The model under review builds one solid part; all positions refer to its coordinate system, in mm. Coordinates: 2 decimals unless noted, no trailing zeros. Loops run counter-clockwise (first coordinate to the right, second up) from the corner with the lowest first, then second, coordinate; pieces in that order, holes last. Notation, with made-up numbers: (73.5, 46.5) - (93.5, 46.5) arc R18 ccw to (93.5, 61.5) - close; hole circle Ø11 at (-31.75, -31.5). An arc over 180 degrees is marked (long way). Answer in a Markdown table with one row per item. Add a question column.
(1) We need section A-A on y = 108.5. Write out the cut boundary in (x, z).
(2) For P1, Ø6, axis at x = -1, y = 113.5, coming from the +Z side; P2, Ø1.5, axis at y = 102.5, z = -5.5, coming from the +X side; P3, Ø8, axis at y = 82, z = 4.5, coming from the +X side; P4, Ø8, axis at x = 0, z = 0, coming from the -Y side, all flat-tipped, find the tip position at first contact; note any pin that passes through.
(3) We need section B-B on y = 37. Write out the cut boundary in (x, z).
(4) For line 1 along X through (y, z) = (10.5, 0); line 2 along Y through (x, z) = (-6, 2.25); line 3 along Z through (x, y) = (2.5, 11), list the stretches that pass through material, from the lowest coordinate up.
(5) Mouldability with a two-part tool opening along X and no side actions: class faces 1 (the cylindrical face through (0.59, 7.6, 4.46)), 2 (the flat face through (-3, 98.298, 3)), 3 (the cylindrical face through (-3.843, 113.951, -0.853)), 4 (the conical face through (-0.169, 17.234, -0.763)) as +X half, -X half, draft (parallel to the pull), parting line (faces both ways), or undercut.
from build123d import *

# Parameters (mm, degrees)
SKETCH1_R                  = 7.14375
BOSS_EXTRUDE1_DEPTH        = 130.048
M10X1_0_TAPPED_HOLE1_D     = 9
M10X1_0_TAPPED_HOLE1_DEPTH = 15
M10X1_0_TAPPED_HOLE1_TIP   = 2.703872786
CUT_EXTRUDE1_START         = -31.75
SKETCH4_R                  = 7.14375
SKETCH4_R_2                = 3.937
CUT_EXTRUDE1_DEPTH         = 31.75


with BuildPart() as part:
    # Sketch1 → Boss-Extrude1 (new body)
    with BuildSketch(Plane(origin=(0, 0, 0), x_dir=(1, 0, 0), z_dir=(0, 1, 0))):
        with Locations(Location((0, 0, 0), (0, 0, 270))):
            Circle(SKETCH1_R)
    extrude(amount=BOSS_EXTRUDE1_DEPTH)

    # M10x1.0 Tapped Hole1
    with Locations(Plane.XZ):
        with Locations((0, 0)):
            Hole(M10X1_0_TAPPED_HOLE1_D / 2, depth=M10X1_0_TAPPED_HOLE1_DEPTH)
            with Locations((0, 0, -(M10X1_0_TAPPED_HOLE1_DEPTH + M10X1_0_TAPPED_HOLE1_TIP / 2))):  # 118° drill point
                Cone(0, M10X1_0_TAPPED_HOLE1_D / 2, M10X1_0_TAPPED_HOLE1_TIP, mode=Mode.SUBTRACT)

    # Sketch4 → Cut-Extrude1 (cut)
    with BuildSketch(Plane(origin=(0, 130.048, 0), x_dir=(1, 0, 0), z_dir=(0, 1, 0)).offset(CUT_EXTRUDE1_START)):
        with Locations(Location((0, 0, 0), (0, 0, 270))):
            Circle(SKETCH4_R)
        with Locations(Location((0, 0, 0), (0, 0, 270))):
            Circle(SKETCH4_R_2, mode=Mode.SUBTRACT)
    extrude(amount=CUT_EXTRUDE1_DEPTH, mode=Mode.SUBTRACT)


solid = part.part
Outcome:
| question | item | result |
|---|---|---|
| 1 | outline | circle Ø7.87 at (0, 0) |
| 2 | P1 | z = 3.94 |
| 2 | P2 | through |
| 2 | P3 | x = 7.13 |
| 2 | P4 | y = 15.3 |
| 3 | outline | circle Ø14.29 at (0, 0) |
| 4 | line 1 | -7.14 to -4.5, 4.5 to 7.14 |
| 4 | line 2 | 0 to 98.3 |
| 4 | line 3 | -6.69 to -3.74, 3.74 to 6.69 |
| 5 | face 1 | undercut |
| 5 | face 2 | draft |
| 5 | face 3 | parting line |
| 5 | face 4 | undercut |
